from build123d import *

# Parameters (mm, degrees)
BOSS_EXTRUDE1_DEPTH   = 52
SKETCH2_R             = 1.7
SKETCH2_W             = 8
SKETCH2_H             = 2
CUT_EXTRUDE1_DEPTH    = 52
SKETCH3_R             = 3.25
CUT_EXTRUDE2_DEPTH    = 3
SKETCH4_R             = 1.9780711
CUT_EXTRUDE3_DEPTH    = 15.5
M4_TAPPED_HOLE1_D     = 3.3
M4_TAPPED_HOLE1_DEPTH = 10.1
M4_TAPPED_HOLE1_TIP   = 0.991420021
SKETCH7_W             = 40
SKETCH7_H             = 3
CUT_EXTRUDE4_DEPTH    = 51
M3_TAPPED_HOLE1_D     = 2.5
M3_TAPPED_HOLE1_DEPTH = 7.5
M3_TAPPED_HOLE1_TIP   = 0.751075774
M3_TAPPED_HOLE2_D     = 2.5
M3_TAPPED_HOLE2_DEPTH = 7.5
M3_TAPPED_HOLE2_TIP   = 0.751075774


with BuildPart() as part:
    # Sketch1 → Boss-Extrude1 (new body)
    with BuildSketch(Plane.XY):
        Polygon((-25.815712776, -13.506468073), (28.984287224, -13.506468073), (28.984287224, -24.506468073), (30.484287224, -24.506468073), (30.484287224, -24.006468073), (44.184287224, -24.006468073), (44.184287224, -33.506468073), (24.184287224, -33.506468073), (24.184287224, -38.506468073), (-25.815712776, -38.506468073), align=None)
    extrude(amount=BOSS_EXTRUDE1_DEPTH)

    # Sketch2 → Cut-Extrude1 (cut)
    with BuildSketch(Plane(origin=(0, -13.506468073, 0), x_dir=(1, 0, 0), z_dir=(0, 1, 0))):
        with Locations((-5.815712776, -12)):
            Circle(SKETCH2_R)
        with Locations((9.184287224, -12)):
            Circle(SKETCH2_R)
        with Locations((-5.815712776, -40)):
            Circle(SKETCH2_R)
        with Locations((9.184287224, -40)):
            Circle(SKETCH2_R)
        with Locations((-16.315712776, -51)):
            Rectangle(SKETCH2_W, SKETCH2_H)
        with Locations((-16.315712776, -1)):
            Rectangle(SKETCH2_W, SKETCH2_H)
        Polygon((-22.815712776, -23.3), (-25.815712776, -23.3), (-25.815712776, -28.3), (-22.815712776, -28.3), (-22.815712776, -30), (-18.815712776, -30), (-18.815712776, -22), (-22.815712776, -22), align=None)
    extrude(amount=-CUT_EXTRUDE1_DEPTH, mode=Mode.SUBTRACT)

    # Sketch3 → Cut-Extrude2 (cut)
    with BuildSketch(Plane(origin=(0, -13.506468073, 0), x_dir=(1, 0, 0), z_dir=(0, 1, 0))):
        with Locations((-5.815712776, -12)):
            Circle(SKETCH3_R)
        with Locations((9.184287224, -12)):
            Circle(SKETCH3_R)
        with Locations((9.184287224, -40)):
            Circle(SKETCH3_R)
        with Locations((-5.815712776, -40)):
            Circle(SKETCH3_R)
    extrude(amount=-CUT_EXTRUDE2_DEPTH, mode=Mode.SUBTRACT)

    # Sketch4 → Cut-Extrude3 (cut, through all)
    with BuildSketch(Plane(origin=(0, -24.006468073, 0), x_dir=(1, 0, 0), z_dir=(0, 1, 0))):
        with Locations((32.184287224, -26)):
            Circle(SKETCH4_R)
    extrude(amount=-CUT_EXTRUDE3_DEPTH, mode=Mode.SUBTRACT)

    # M4 Tapped Hole1
    with Locations(Plane(origin=(0, -24.006468073, 0), x_dir=(1, 0, 0), z_dir=(0, 1, 0))):
        with Locations((34.600682557, -6), (34.600682557, -16), (34.600682557, -36), (34.600682557, -46)):
            Hole(M4_TAPPED_HOLE1_D / 2, depth=M4_TAPPED_HOLE1_DEPTH)
            with Locations((0, 0, -(M4_TAPPED_HOLE1_DEPTH + M4_TAPPED_HOLE1_TIP / 2))):  # 118° drill point
                Cone(0, M4_TAPPED_HOLE1_D / 2, M4_TAPPED_HOLE1_TIP, mode=Mode.SUBTRACT)

    # Sketch7 → Cut-Extrude4 (cut, through all)
    with BuildSketch(Plane(origin=(24.184287224, 0, 0), x_dir=(0, 0, -1), z_dir=(1, 0, 0))):
        with Locations((-26, -37.006468073)):
            Rectangle(SKETCH7_W, SKETCH7_H)
    extrude(amount=-CUT_EXTRUDE4_DEPTH, mode=Mode.SUBTRACT)

    # M3 Tapped Hole1
    with Locations(Plane.XY.offset(50)):
        with Locations((-16.315712776, -18.506468073), (-16.315712776, -30.506468073)):
            Hole(M3_TAPPED_HOLE1_D / 2, depth=M3_TAPPED_HOLE1_DEPTH)
            with Locations((0, 0, -(M3_TAPPED_HOLE1_DEPTH + M3_TAPPED_HOLE1_TIP / 2))):  # 118° drill point
                Cone(0, M3_TAPPED_HOLE1_D / 2, M3_TAPPED_HOLE1_TIP, mode=Mode.SUBTRACT)

    # M3 Tapped Hole2
    with Locations(Plane(origin=(0, 0, 2), x_dir=(-1, 0, 0), z_dir=(0, 0, -1))):
        with Locations((16.315712776, -18.506468073), (16.315712776, -30.506468073)):
            Hole(M3_TAPPED_HOLE2_D / 2, depth=M3_TAPPED_HOLE2_DEPTH)
            with Locations((0, 0, -(M3_TAPPED_HOLE2_DEPTH + M3_TAPPED_HOLE2_TIP / 2))):  # 118° drill point
                Cone(0, M3_TAPPED_HOLE2_D / 2, M3_TAPPED_HOLE2_TIP, mode=Mode.SUBTRACT)


solid = part.part
For this review, take the finished solid that the model builds, in its own axes (mm). A direction names the side the tool comes from. Coordinates: 2 decimals unless noted, no trailing zeros. Loops run counter-clockwise (first coordinate to the right, second up) from the corner with the lowest first, then second, coordinate; pieces in that order, holes last. Notation, with made-up numbers: (42.25, -28) - (97.25, -28) arc R24 ccw to (97.25, -5) - close; hole circle Ø4 at (85.25, 60.5). An arc over 180 degrees is marked (long way). Return JSON: item names as keys, results as strings.
Item 1: Take a section at C-C (z = 12). Give the boundary of the cut face in (x, y), then the cut area to 3 significant figures.
Determined:
{"outline": "(-25.82, -35.51) - (-7.52, -35.51) - (-7.52, -16.51) - (-9.07, -16.51) - (-9.07, -13.51) - (-25.82, -13.51) - close; (-4.12, -35.51) - (7.48, -35.51) - (7.48, -16.51) - (5.93, -16.51) - (5.93, -13.51) - (-2.57, -13.51) - (-2.57, -16.51) - (-4.12, -16.51) - close; (10.88, -35.51) - (24.18, -35.51) - (24.18, -33.51) - (44.18, -33.51) - (44.18, -24.01) - (30.48, -24.01) - (30.48, -24.51) - (28.98, -24.51) - (28.98, -13.51) - (12.43, -13.51) - (12.43, -16.51) - (10.88, -16.51) - close", "area": "1,170 mm2"}
Item 2: For faces 1 (the cylindrical face through (8.48, -14.985, 43.173)), 2 (the flat face through (0, -37, 6)), 3 (the cylindrical face through (-16.893, -31.615, 46.198)), 4 (the flat face through (-12.316, -26, 51)), list the 3-axis set-ups (+Z, -Z, +X, -X, +Y, -Y) from which the entire face can be reached by the end or side of a thin tool; tool diameter is ignored.
Determined:
{"face 1": "+Y", "face 2": "+X, -X, -Y", "face 3": "+Z", "face 4": "+Z, +Y, -Y"}
Item 3: Mouldability with a two-part tool opening along Z and no side actions: class faces 5 (the flat face through (-20.316, -26, 1)), 6 (the conical face through (-16.29, -18.29, 10.12)), 7 (the flat face through (-24, -24, 28.3)), 8 (the cylindrical face through (-4.07, -14.99, 9.26)) as pulls with the +Z half, pulls with the -Z half, needs draft (parallel to the pull), parting line crosses it, or undercut.
Determined:
{"face 5": "needs draft", "face 6": "pulls with the -Z half", "face 7": "undercut", "face 8": "undercut"}
Item 4: Take a section at A-A (z = 36). Give the boundary of the cut face in (x, y), then the cut area to 3 significant figures.
Determined:
{"outline": "(-25.82, -35.51) - (24.18, -35.51) - (24.18, -33.51) - (32.95, -33.51) - (32.95, -24.01) - (30.48, -24.01) - (30.48, -24.51) - (28.98, -24.51) - (28.98, -13.51) - (-25.82, -13.51) - close; (36.25, -33.51) - (44.18, -33.51) - (44.18, -24.01) - (36.25, -24.01) - close", "area": "1,310 mm2"}
Item 5: For line 1 (X direction, y = -28.75, z = 36); line 2 (Z direction, x = 7.5, y = -35.75); line 3 (Z direction, x = -7, y = -15.5), list the stretches that pass through material, from the lowest coordinate up.
Determined:
{"line 1": "x = -25.82 to 32.95, 36.25 to 44.18", "line 2": "z = 0 to 6, 46 to 52", "line 3": "z = 0 to 8.97, 15.03 to 36.97, 43.03 to 52"}
Item 6: Take a section at B-B (y = -21.25). Give the boundary of the cut face in (x, z).
Determined:
{"outline": "(-25.82, 0) - (-20.32, 0) - (-20.32, 2) - (-12.32, 2) - (-12.32, 0) - (28.98, 0) - (28.98, 52) - (-12.32, 52) - (-12.32, 50) - (-20.32, 50) - (-20.32, 52) - (-25.82, 52) - (-25.82, 28.3) - (-22.82, 28.3) - (-22.82, 30) - (-18.82, 30) - (-18.82, 22) - (-22.82, 22) - (-22.82, 23.3) - (-25.82, 23.3) - close; hole circle Ø3.4 at (-5.82, 12); hole circle Ø3.4 at (-5.82, 40); hole circle Ø3.4 at (9.18, 12); hole circle Ø3.4 at (9.18, 40)"}
Item 7: Take a section at D-D (y = -26.5). State how many separate pieces and enclosed holes the cut face has, then the cut area to 3 significant figures.
Determined:
{"separate pieces": "1", "enclosed holes": "9", "area": "3,480 mm2"}
Item 8: Insertion check: pin 1 (15 mm diameter, centred on x = 37, z = 16.5, fed in from +Y); pin 2 (6.5 mm diameter, centred on x = 32.18, z = 26, fed in from -Y); pin 3 (3 mm diameter, centred on x = 23, z = 38, fed in from -Y). Each pin has a flat end and moves straight along its axis. Give the tip position at first contact, or say it passes through.
Determined:
{"pin 1": "stops at y = -24.01", "pin 2": "stops at y = -33.51", "pin 3": "stops at y = -35.51"}
